```python
from build123d import *

# Parameters (mm, degrees)
F0_W     = 127
F0_H     = 127
F1_DEPTH = 127
F3_DEPTH = 6.35
F4_W     = 101.6
F4_H     = 101.6
F5_DEPTH = 127


with BuildPart() as f1:
    # F0 (on Top) → F1 (new body)
    with BuildSketch(Plane.XY):
        Rectangle(F0_W, F0_H)
    extrude(amount=F1_DEPTH)

    # F2 (on face) → F3 (cut)
    with BuildSketch(Plane.XY.offset(127)):
        with BuildLine():
            Line((-50.8, -57.15), (50.8, -57.15))
            ThreePointArc((50.8, -57.15), (55.290128, -55.290128), (57.15, -50.8))
            Line((57.15, -50.8), (57.15, 50.8))
            ThreePointArc((57.15, 50.8), (55.290128, 55.290128), (50.8, 57.15))
            Line((50.8, 57.15), (-50.8, 57.15))
            ThreePointArc((-50.8, 57.15), (-55.290128, 55.290128), (-57.15, 50.8))
            Line((-57.15, 50.8), (-57.15, -50.8))
            ThreePointArc((-57.15, -50.8), (-55.290128, -55.290128), (-50.8, -57.15))
        make_face()
    extrude(amount=-F3_DEPTH, mode=Mode.SUBTRACT)

    # F4 (on face) → F5 (cut)
    with BuildSketch(Plane.XY.offset(120.65)):
        Rectangle(F4_W, F4_H)
    extrude(amount=-F5_DEPTH, mode=Mode.SUBTRACT)


solid = f1.part
```
The listing builds one solid part. Answer for the finished solid, in the listing's coordinates (mm). A direction names the side the tool comes from. Give positions to 0.01 mm unless a question says otherwise; leave off trailing zeros. Order: outer loops, then holes, each group sorted by start corner. A loop starts at its lowest first (then second) coordinate and runs counter-clockwise, first axis right, second up. Notation, with made-up numbers: M 30.25,-2.5 L 59.25,-2.5 A16 ccw 59.25,6.5 Z; hole C 30.5,24 d1. An arc over 180 degrees is marked long. Put each result on its own line as item: value. Start each with the question number.
Item 1: The part is cut by section D-D, the plane y = -54. Determine the outline of the cut face in (x, z), and give its area (3 significant figures).
Item 2: For a pull along Y with two mould halves and no side action, classify faces 1 (the face through (-63.5, -1, 63)), 2 (the face through (-1, 63.5, 63)), 3 (the face through (-57.15, 1, 124)) as +Y half, -Y half, draft (parallel to the pull), parting line (faces both ways), or undercut.
Item 3: The part is cut by section C-C, the plane z = 100. Determine the outline of the cut face in (x, y).
Item 4: The part is cut by section A-A, the plane x = 24.5. Determine the outline of the cut face in (y, z).
Item 5: Which of the six approach directions +Z, -Z, +X, -X, +Y, -Y give full straight-line access (tool end or side, diameter ignored) to faces 4 (the face through (-1, -63.5, 63)), 5 (the face through (-50.8, -1, 61)), 6 (the face through (55.34, 55.24, 123.87))?
Item 6: Find the intervals of material crossed by line 1 along Y through (x, z) = (-10, 74.5); line 2 along Z through (x, y) = (-57, -37), in increasing order.
Answer key:
1. outline: M -63.5,0 L 63.5,0 L 63.5,127 L 56.28,127 L 56.28,120.65 L -56.28,120.65 L -56.28,127 L -63.5,127 Z
1. area: 15,400 mm²
2. face 1: draft
2. face 2: +Y half
2. face 3: undercut
3. outline: M -63.5,-63.5 L 63.5,-63.5 L 63.5,63.5 L -63.5,63.5 Z; hole M -50.8,-50.8 L 50.8,-50.8 L 50.8,50.8 L -50.8,50.8 Z
4. outline: M -63.5,0 L -50.8,0 L -50.8,120.65 L -57.15,120.65 L -57.15,127 L -63.5,127 Z; M 50.8,0 L 63.5,0 L 63.5,127 L 57.15,127 L 57.15,120.65 L 50.8,120.65 Z
5. face 4: +Z, -Z, +X, -X, -Y
5. face 5: +Z, -Z
5. face 6: +Z
6. line 1: y = -63.5 to -50.8, 50.8 to 63.5
6. line 2: z = 0 to 120.65
